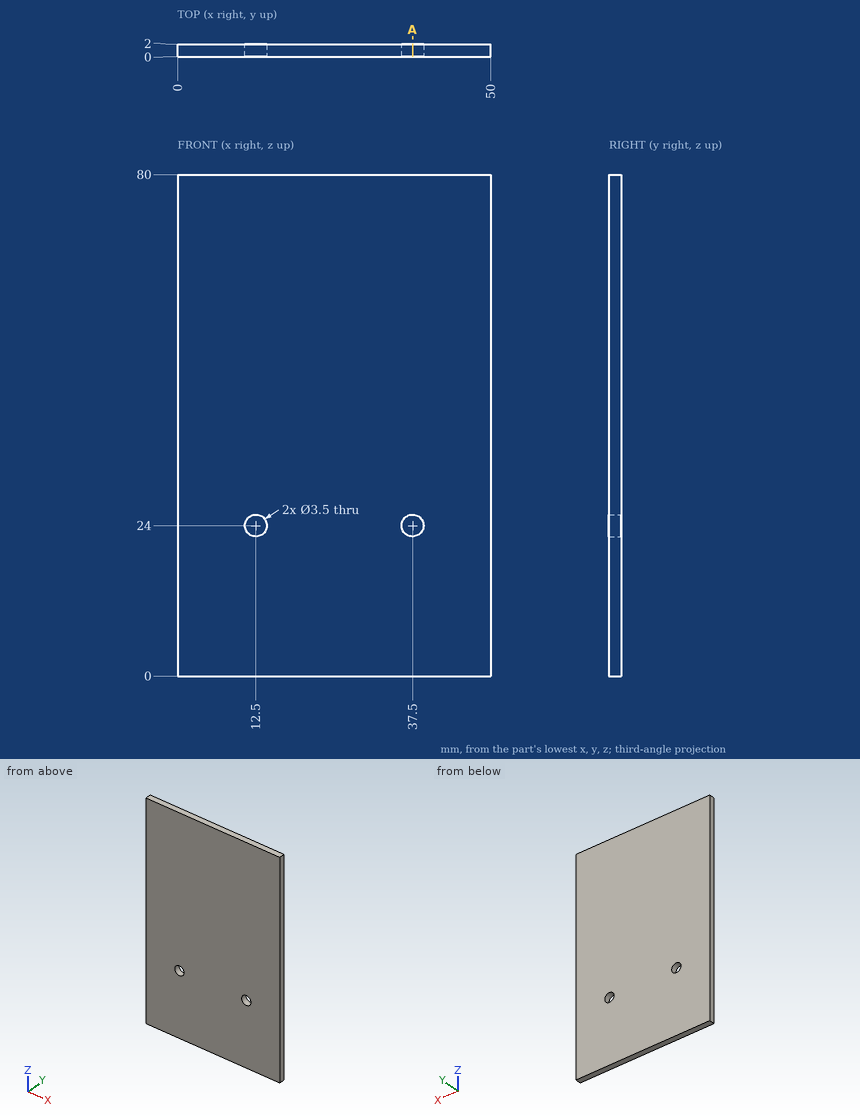
Check sheet for the drawn part. Datum: minimum x, y, z corner. Units: mm. Round coordinates to 2 decimals unless told otherwise and drop trailing zeros. Order: outer loops, then holes, each group sorted by start corner. A loop starts at its lowest first (then second) coordinate and runs counter-clockwise, first axis right, second up.
1. Section check A-A on x = 37.5. Record the cut outline in (y, z), then the cut area to 3 significant figures.
Final values:
outline: (0, 0) - (2, 0) - (2, 22.25) - (0, 22.25) - close; (0, 25.75) - (2, 25.75) - (2, 80) - (0, 80) - close
area: 153 mm2
2. Go/stop test with flat-tipped pins: P1, Ø5, axis at x = 25.5, z = 31.5, coming from the -Y side; P2, Ø3, axis at x = 37.5, z = 24, coming from the +Y side. Record where each tip stops, or that it passes through.
Final values:
P1: stops at y = 0
P2: passes through
3. Thickness scan on L1, parallel to X at y = 0.7, z = 24; L2, parallel to Z at x = 12.5, y = 1.45; L3, parallel to Z at x = 11, y = 0.75. Record the ranges inside material, lowest first.
Final values:
L1: x = 0 to 10.75, 14.25 to 35.75, 39.25 to 50
L2: z = 0 to 22.25, 25.75 to 80
L3: z = 0 to 23.1, 24.9 to 80
